Work out the finished part from the listing and answer in its coordinate system (mm). Give positions to 0.01 mm unless a question says otherwise; leave off trailing zeros. Order: outer loops, then holes, each group sorted by start corner. A loop starts at its lowest first (then second) coordinate and runs counter-clockwise, first axis right, second up.
```python
from build123d import *

# Parameters (mm, degrees)
SKETCH_1_R          = 7
EXTRUDE_1_DEPTH     = 9
SKETCH_2_W          = 2
SKETCH_2_H          = 2
EXTRUDE_2_DEPTH     = 45
CUT_EXTRUDE_1_DEPTH = 4
SKETCH_5_W          = 2
SKETCH_5_H          = 2
EXTRUDE_3_DEPTH     = 4


with BuildPart() as part:
    # 草图1 → 凸台-拉伸1 (new body)
    with BuildSketch(Plane.XY):
        Circle(SKETCH_1_R)
    extrude(amount=EXTRUDE_1_DEPTH)

    # 草图2 → 凸台-拉伸2 (add)
    with BuildSketch(Plane.XY.offset(9)):
        with Locations((3.25, 3.25)):
            Rectangle(SKETCH_2_W, SKETCH_2_H)
        with Locations((-3.25, 3.25)):
            Rectangle(SKETCH_2_W, SKETCH_2_H)
        with Locations((3.25, -3.25)):
            Rectangle(SKETCH_2_W, SKETCH_2_H)
        with Locations((-3.25, -3.25)):
            Rectangle(SKETCH_2_W, SKETCH_2_H)
    extrude(amount=EXTRUDE_2_DEPTH)

    # 草图4 → 切除-拉伸1 (cut)
    with BuildSketch(Plane(origin=(0, 0, 0), x_dir=(-1, 0, 0), z_dir=(0, 0, -1))):
        Polygon((-2.500889242, 1.671040767), (-2.95, 1.221930009), (-2.95, 0.586791484), (-3.193056991, 0), (-2.95, -0.586791484), (-2.95, -1.221930009), (-2.500889242, -1.671040767), (-2.257832251, -2.257832251), (-1.671040767, -2.500889242), (-1.221930009, -2.95), (-0.586791484, -2.95), (0, -3.193056991), (0.586791484, -2.95), (1.221930009, -2.95), (1.671040767, -2.500889242), (2.257832251, -2.257832251), (2.500889242, -1.671040767), (2.95, -1.221930009), (2.95, -0.586791484), (3.193056991, 0), (2.95, 0.586791484), (2.95, 1.221930009), (2.500889242, 1.671040767), (2.257832251, 2.257832251), (1.671040767, 2.500889242), (1.221930009, 2.95), (0.586791484, 2.95), (0, 3.193056991), (-0.586791484, 2.95), (-1.221930009, 2.95), (-1.671040767, 2.500889242), (-2.257832251, 2.257832251), align=None)
    extrude(amount=-CUT_EXTRUDE_1_DEPTH, mode=Mode.SUBTRACT)

    # 草图5 → 凸台-拉伸3 (add)
    with BuildSketch(Plane(origin=(0, 0, 4), x_dir=(-1, 0, 0), z_dir=(0, 0, -1))):
        Rectangle(SKETCH_5_W, SKETCH_5_H)
    extrude(amount=EXTRUDE_3_DEPTH)


solid = part.part
```
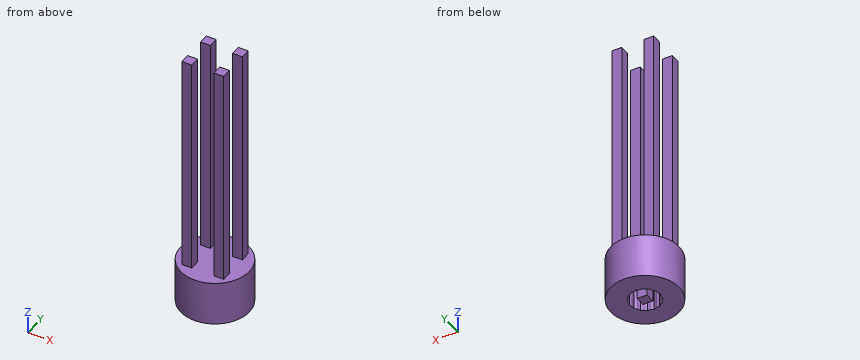
1. Straight lines are drawn through the part: probe 1 along X at (y, z) = (-3.25, 20.5); probe 2 along Z at (x, y) = (-5, -3.75). For each, find the intervals that lie inside material, in ascending order.
Findings below:
probe 1: x = -4.25 to -2.25, 2.25 to 4.25
probe 2: z = 0 to 9
2. Given P1, Ø1, axis at y = -3, z = 32.5, coming from the -X side; P2, Ø2, axis at y = 3.5, z = 26.5, coming from the +X side; P3, Ø0.7, axis at y = -1, z = 2, coming from the +X side, each flat-ended and moving along its own axis, determine where each tip first touches the part or whether it passes through.
Findings below:
P1: stops at x = -4.25
P2: stops at x = 4.25
P3: stops at x = 6.97
3. The part is cut by section A-A (z = 41). Write down the section's boundary in (x, y).
Findings below:
outline: (-4.25, -4.25) - (-2.25, -4.25) - (-2.25, -2.25) - (-4.25, -2.25) - close; (-4.25, 2.25) - (-2.25, 2.25) - (-2.25, 4.25) - (-4.25, 4.25) - close; (2.25, -4.25) - (4.25, -4.25) - (4.25, -2.25) - (2.25, -2.25) - close; (2.25, 2.25) - (4.25, 2.25) - (4.25, 4.25) - (2.25, 4.25) - close
4. The part is cut by section B-B (y = 3.75). Write down the section's boundary in (x, z).
Findings below:
outline: (-5.91, 0) - (5.91, 0) - (5.91, 9) - (4.25, 9) - (4.25, 54) - (2.25, 54) - (2.25, 9) - (-2.25, 9) - (-2.25, 54) - (-4.25, 54) - (-4.25, 9) - (-5.91, 9) - close
